Can you work these out from the model? Positions are in its coordinate system, mm. Face numbers are marked on the shaded views. Give positions to 0.01 mm unless a question says otherwise; leave off trailing zeros. Loops run counter-clockwise (first coordinate to the right, second up) from the corner with the lowest first, then second, coordinate; pieces in that order, holes last. Notation, with made-up numbers: (-10.75, -1) -> (34.25, -1) arc R20 ccw to (34.25, 17) -> close; hole circle Ø3 at (71.25, 35). An arc over 180 degrees is marked (long way). Use CSV: the item, a comma, the result in double quotes.
from build123d import *

# Parameters (mm, degrees)
SKETCH1_R           = 15
SKETCH1_R_2         = 10
BOSS_EXTRUDE1_DEPTH = 30
SKETCH2_W           = 50
SKETCH2_H           = 50
BOSS_EXTRUDE2_DEPTH = 10
SKETCH3_R           = 2.5
CUT_EXTRUDE1_DEPTH  = 10
SKETCH4_R           = 15
SKETCH4_R_2         = 10
CUT_EXTRUDE2_DEPTH  = 30
SKETCH5_R           = 15
CUT_EXTRUDE3_DEPTH  = 30


with BuildPart() as part:
    # Sketch1 → Boss-Extrude1 (new body)
    with BuildSketch(Plane.XY):
        Circle(SKETCH1_R)
        Circle(SKETCH1_R_2, mode=Mode.SUBTRACT)
    extrude(amount=BOSS_EXTRUDE1_DEPTH)

    # Sketch2 → Boss-Extrude2 (add)
    with BuildSketch(Plane(origin=(0, 0, 0), x_dir=(-1, 0, 0), z_dir=(0, 0, -1))):
        Rectangle(SKETCH2_W, SKETCH2_H)
    extrude(amount=BOSS_EXTRUDE2_DEPTH)

    # Sketch3 → Cut-Extrude1 (cut)
    with BuildSketch(Plane.XY):
        with Locations((-17.5, 17.5)):
            Circle(SKETCH3_R)
        with Locations((-17.5, -17.5)):
            Circle(SKETCH3_R)
        with Locations((17.5, -17.5)):
            Circle(SKETCH3_R)
        with Locations((17.5, 17.5)):
            Circle(SKETCH3_R)
    extrude(amount=-CUT_EXTRUDE1_DEPTH, mode=Mode.SUBTRACT)

    # Sketch4 → Cut-Extrude2 (cut)
    with BuildSketch(Plane.XY):
        Circle(SKETCH4_R)
        Circle(SKETCH4_R_2, mode=Mode.SUBTRACT)
    extrude(amount=CUT_EXTRUDE2_DEPTH, mode=Mode.SUBTRACT)

    # Sketch5 → Cut-Extrude3 (cut)
    with BuildSketch(Plane.XY):
        Circle(SKETCH5_R)
    extrude(amount=-CUT_EXTRUDE3_DEPTH, mode=Mode.SUBTRACT)


solid = part.part
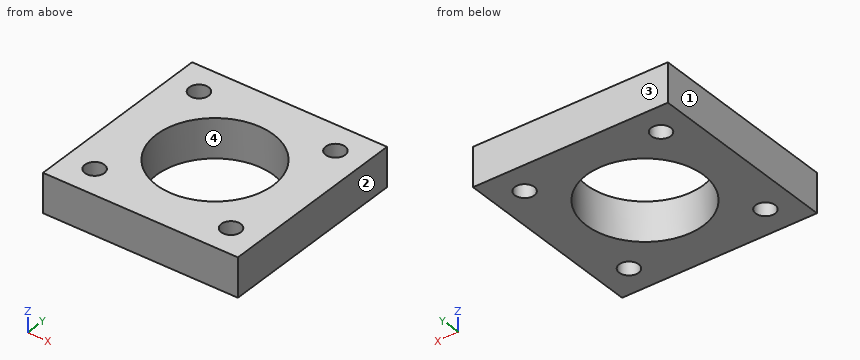
(1) If we section it at B-B, the plane x = 12: Write out the boundary of the cut face in (y, z), then the cut area to 3 significant figures.
Answer sheet:
outline,"(-25, -10) -> (-9, -10) -> (-9, 0) -> (-25, 0) -> close; (9, -10) -> (25, -10) -> (25, 0) -> (9, 0) -> close"
area,"320 mm2"
(2) If I drill on L1, parallel to Y at x = 17.5, z = -8; L2, parallel to X at y = 0.5, z = -2.5; L3, parallel to Y at x = 0, z = -5.75, over which ranges is the centre line in solid material (lowest first)? Write a range as from..to.
Answer sheet:
L1,"y = -25..-20, -15..15, 20..25"
L2,"x = -25..-14.99, 14.99..25"
L3,"y = -25..-15, 15..25"
(3) We'd pull the mould along X, two halves only. Please class the marked faces 1, 2, 3 and 4: released by +X, released by -X, zero draft, split by the parting line, or undercut.
Answer sheet:
face 1,"released by -X"
face 2,"released by +X"
face 3,"zero draft"
face 4,"undercut"
(4) Will this pin go through, and if not, where does the flat tip stop? pin 1 Ø10 at (x, y) = (-5, -13.5) entering from -Z.
Answer sheet:
pin 1,"stops at z = -10"
(5) If we section it at A-A, the plane y = 17.5: Write out the boundary of the cut face in (x, z).
Answer sheet:
outline,"(-25, -10) -> (-20, -10) -> (-20, 0) -> (-25, 0) -> close; (-15, -10) -> (15, -10) -> (15, 0) -> (-15, 0) -> close; (20, -10) -> (25, -10) -> (25, 0) -> (20, 0) -> close"
